Part model, mm, in its own coordinate system. A direction names the side the tool comes from. Give positions to 0.01 mm unless a question says otherwise; leave off trailing zeros. Order: outer loops, then holes, each group sorted by start corner. A loop starts at its lowest first (then second) coordinate and runs counter-clockwise, first axis right, second up. Notation, with made-up numbers: M 83.25,88.5 L 130.25,88.5 A23 ccw 130.25,105.5 Z; hole C 41,39 d1. An arc over 180 degrees is marked long. Answer as a JSON object with one key per item and string values.
Autodesk Inventor part; units mm, degrees
ref_plane "Work Plane2" through (0, 0, 0) normal (0, 0, 1) x (1, 0, 0)
ref_plane "YZ Plane" through (0, 0, 0) normal (1, 0, 0) x (0, 1, 0)
ref_plane "XZ Plane" through (0, 0, 0) normal (0, 1, 0) x (-1, 0, 0)
sketch "Sketch1" plane through (0, 0, 0) normal (0, 0, 1) x (1, 0, 0)
  line L0 (-2, 3.4641) -> (2, 3.4641)
  line L1 (-4, 0) -> (-2, 3.4641)
  line L2 (-2, -3.4641) -> (-4, 0)
  line L3 (2, -3.4641) -> (-2, -3.4641)
  line L4 (4, 0) -> (2, -3.4641)
  line L5 (2, 3.4641) -> (4, 0)
  line L6 (-4, 0) -> (-2, 3.4641)
  line L7 (-2, 3.4641) -> (2, 3.4641)
  line L8 (2, 3.4641) -> (4, 0)
  line L9 (4, 0) -> (2, -3.4641)
  line L10 (2, -3.4641) -> (-2, -3.4641)
  line L11 (-2, -3.4641) -> (-4, 0)
  circle A0 centre (0, 0) radius 7.5
  circle A1 centre (0, 0) radius 6.5
  point P0 (0, 0)
  dimension "d0" = 1
extrude "Extrusion1" add sketch "Sketch1" against normal blind 10 contours L0 L5 L4 L3 L2 L1
ref_plane "Work Plane2" through (0, 0, 0) normal (0, 0, 1) x (1, 0, 0)
sketch "Sketch3" plane through (0, 0, 0) normal (0, 0, 1) x (1, 0, 0)
  circle A0 centre (0, 0) radius 6.5
  point P0 (0, 0)
extrude "Extrusion2" add sketch "Sketch3" along normal blind 2
sketch "Sketch4" plane through (0, 0, 2) normal (0, 0, 1) x (1, 0, 0)
  circle A0 centre (0, 0) radius 17.25
  circle A1 centre (0, 0) radius 14.45 construction
  point P0 (14.45, 0)
  point P1 (-14.45, 0)
  point P2 (0, 14.45)
  point P3 (0, -14.45)
  dimension "d5" = 34.5
  dimension "d6" = 28.9
extrude "Extrusion3" add sketch "Sketch4" along normal blind 5
hole "Hole1" at (14.45, 0, 2) at (-14.45, 0, 2) at (0, 14.45, 2) at (0, -14.45, 2) direction (0, 0, 1) diameter 1.6 end through all
properties part number "Exagono"
1. Which spindle directions (+Z, -Z, +X, -X, +Y, -Y) get a long thin tool onto all of the face, cutting with end or side? Do faces 4 (the flat face through (0, 3.464, -5)), 5 (the flat face through (-2.986, -1.756, -4.93)), 6 (the flat face through (3, -3, 0)). Say none if no direction does.
Worked answers:
{"face 4": "-Z, +X, -X, +Y", "face 5": "-Z, -X, -Y", "face 6": "-Z"}
2. Cut at B-B on z = 5.5. Give the cut face in (x, y).
Worked answers:
{"outline": "C 0,0 d34.5; hole C -14.45,0 d1.6; hole C 0,-14.45 d1.6; hole C 0,14.45 d1.6; hole C 14.45,0 d1.6"}
3. Probe line 1 along X through (y, z) = (0.5, 3.5); line 2 along Z through (x, y) = (-6, 15); line 3 along Y through (x, z) = (14.45, 5.55). List the from-to ranges inside material, lowest first.
Worked answers:
{"line 1": "x = -17.24 to -15.07, -13.83 to 13.83, 15.07 to 17.24", "line 2": "z = 2 to 7", "line 3": "y = -9.42 to -0.8, 0.8 to 9.42"}
4. Two-plate mould, pull along Y, no slides. Class faces 1 (the cylindrical face through (-0.04, -15.25, 4.54)), 2 (the flat face through (3.014, -1.708, -4.93)), 3 (the cylindrical face through (-5.158, 3.955, 0.986)): +Y half, -Y half, draft (parallel to the pull), parting line (faces both ways), or undercut.
Worked answers:
{"face 1": "undercut", "face 2": "-Y half", "face 3": "parting line"}
5. Cut at A-A on x = 0. Give the cut face in (y, z).
Worked answers:
{"outline": "M -17.25,2 L -15.25,2 L -15.25,7 L -17.25,7 Z; M -13.65,2 L -6.5,2 L -6.5,0 L -3.46,0 L -3.46,-10 L 3.46,-10 L 3.46,0 L 6.5,0 L 6.5,2 L 13.65,2 L 13.65,7 L -13.65,7 Z; M 15.25,2 L 17.25,2 L 17.25,7 L 15.25,7 Z"}
6. Cut at C-C on x = -14.45. Give the cut face in (y, z), plus the area to 3 significant figures.
Worked answers:
{"outline": "M -9.42,2 L -0.8,2 L -0.8,7 L -9.42,7 Z; M 0.8,2 L 9.42,2 L 9.42,7 L 0.8,7 Z", "area": "86.2 mm^2"}
7. Pin check, flat tips, straight feed: P1, Ø1.2, axis at x = 1, z = -6, coming from the +Y side; P2, Ø2, axis at x = -14.45, y = 0, coming from the -Z side; P3, Ø6, axis at y = 1, z = -8, coming from the +X side. Stop position of each tip, or through.
Worked answers:
{"P1": "stops at y = 3.46", "P2": "stops at z = 2", "P3": "stops at x = 4"}
